The drawing under review shows one solid part. Ordinate dimensions are in mm from its lowest x, y, z. A direction names the side the tool comes from. Give positions to 0.01 mm unless a question says otherwise; leave off trailing zeros. Loops run counter-clockwise (first coordinate to the right, second up) from the corner with the lowest first, then second, coordinate; pieces in that order, holes last. Notation, with made-up numbers: M -37.75,-18.5 L -31.75,-18.5 A29 ccw -31.75,20.5 Z; hole C 16,73.5 d11. An arc over 180 degrees is marked long. Answer as CSV lines item,"result".
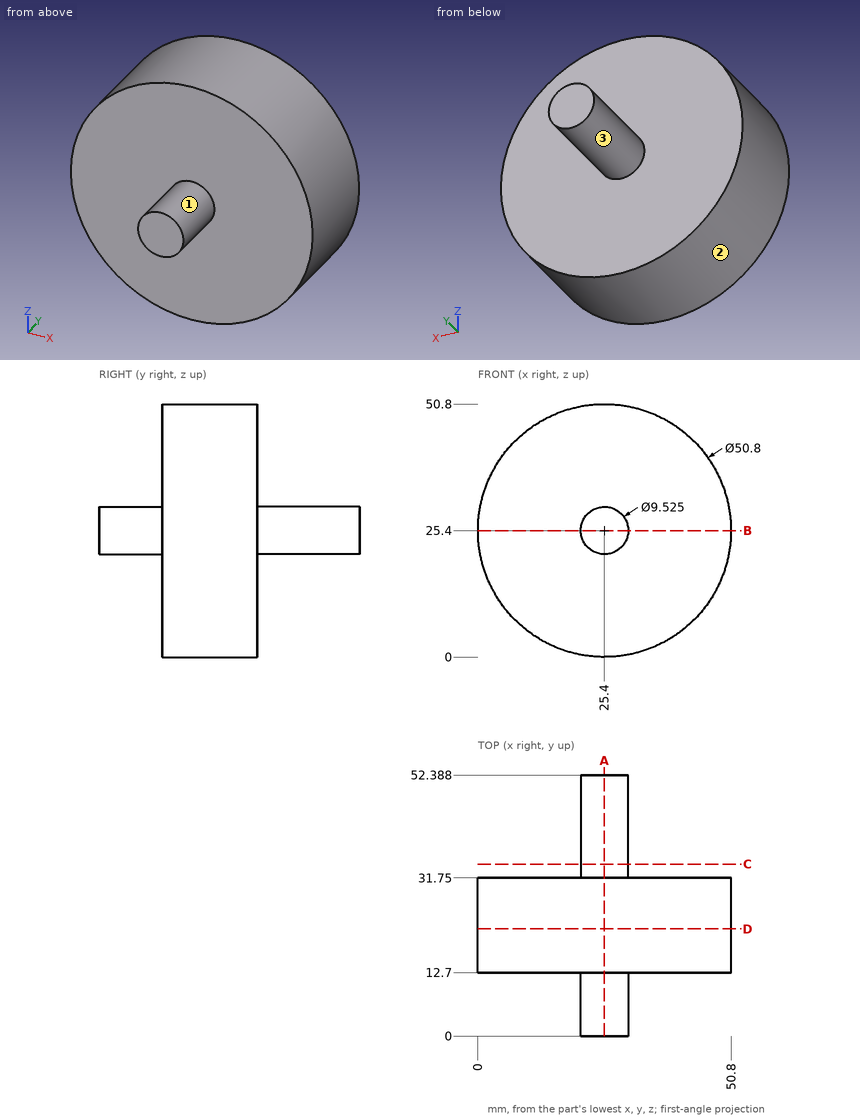
1. To check wall thickness, follow L1, parallel to Y at x = 32.5, z = 9.5; L2, parallel to Z at x = 6, y = 29 (1 decimal); L3, parallel to X at y = 45, z = 21 (1 decimal). State the ranges of each line that lie inside material, in increasing order. Write a range as [from, to].
Answer block:
L1,"[12.7, 31.75]"
L2,"[9, 41.8]"
L3,"[23.6, 27.2]"
2. We need section C-C, the plane y = 34.5. Write out the cut boundary in (x, z) (1 decimal).
Answer block:
outline,"C 25.4,25.4 d9.5"
3. For the marked faces 1, 2 and 3, list the 3-axis set-ups (+Z, -Z, +X, -X, +Y, -Y) from which the entire face can be reached by the end or side of a thin tool; tool diameter is ignored.
Answer block:
face 1,"-Y"
face 2,"+Y, -Y"
face 3,"+Y"
4. We need section D-D, the plane y = 21.5. Write out the cut boundary in (x, z).
Answer block:
outline,"C 25.4,25.4 d50.8"
5. We need section A-A, the plane x = 25.4. Write out the cut boundary in (y, z).
Answer block:
outline,"M 0,20.64 L 12.7,20.64 L 12.7,0 L 31.75,0 L 31.75,20.64 L 52.39,20.64 L 52.39,30.16 L 31.75,30.16 L 31.75,50.8 L 12.7,50.8 L 12.7,30.16 L 0,30.16 Z"
6. For P1, Ø1.5, axis at y = 23.5, z = 45.5, coming from the +X side (1 decimal); P2, Ø2, axis at x = 36.5, z = 43, coming from the +Y side; P3, Ø12, axis at x = 30, y = 12, coming from the +Z side, all flat-tipped, find the tip position at first contact; note any pin that passes through.
Answer block:
P1,"x = 41.9"
P2,"y = 31.75"
P3,"z = 50.8"
7. We need section B-B, the plane z = 25.4. Write out the cut boundary in (x, y), plus the area to 3 significant figures.
Answer block:
outline,"M 0,12.7 L 20.64,12.7 L 20.64,0 L 30.16,0 L 30.16,12.7 L 50.8,12.7 L 50.8,31.75 L 30.16,31.75 L 30.16,52.39 L 20.64,52.39 L 20.64,31.75 L 0,31.75 Z"
area,"1,290 mm²"
